Can you work these out from the model? Positions are in its coordinate system, mm. Coordinates: 2 decimals unless noted, no trailing zeros. Write each loop counter-clockwise with the first axis right and the second up, starting at its lowest first coordinate (ties: lowest second). Pieces come first, ordered by that corner, then holes. Notation, with made-up numbers: (-24.75, 36.25) -> (-17.75, 36.25) arc R28 ccw to (-17.75, 70.25) -> close; hole circle Ø2 at (32, 41). An arc over 180 degrees is marked (long way). Use one line per item in the form item = value.
```python
from build123d import *


with BuildPart() as part:
    # Sketch1 → Revolve1 (revolve)
    with BuildSketch(Plane(origin=(0, 0, 0), x_dir=(0, 0, -1), z_dir=(1, 0, 0)), mode=Mode.PRIVATE) as revolve1_sk:
        with BuildLine():
            Line((0.8, 49), (1.5, 49))
            Line((1.5, 49), (1.5, 46.5))
            Line((1.5, 46.5), (1.25, 46.5))
            Line((1.25, 46.5), (0, 46))
            Line((0, 46), (-1.25, 46.5))
            Line((-1.25, 46.5), (-1.5, 46.5))
            Line((-1.5, 46.5), (-1.5, 49))
            Line((-1.5, 49), (-0.8, 49))
            ThreePointArc((-0.8, 49), (0, 48.833030278), (0.8, 49))
        make_face()
    revolve(revolve1_sk.sketch.rotate(Axis((0, 0, 0), (0, 0, -1)), 90), axis=Axis((0, 0, 0), (0, 0, -1)))


solid = part.part
```
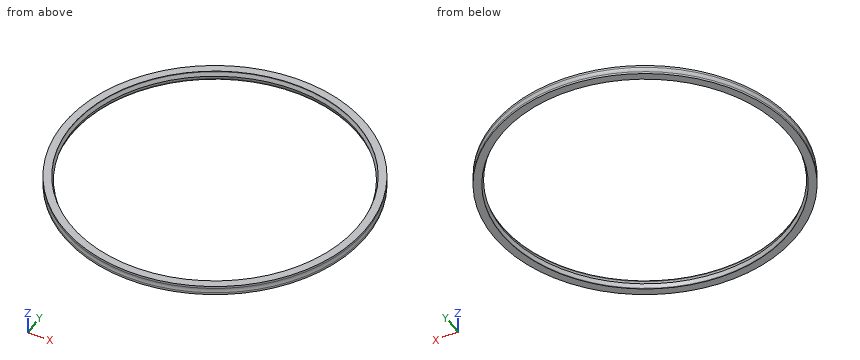
Q1. If I drill on line 1 (Y direction, x = 0, z = -1.25); line 2 (X direction, y = 9.5, z = 1.3); line 3 (Y direction, x = 15, z = -1.3), over which ranges is the centre line in solid material (lowest first)? Write a range as from..to.
Return value:
line_1 = -49..-46.5, 46.5..49
line_2 = -48.07..-45.52, 45.52..48.07
line_3 = -46.65..-44.01, 44.01..46.65
Q2. Will these pins go through, and if not, where does the flat tip stop? pin 1 (1 mm diameter, centred on y = 21.5, z = -1, fed in from +X); pin 2 (12 mm diameter, centred on x = 32, y = 28, fed in from +Z).
Return value:
pin_1 = 44.27
pin_2 = 1.5
Q3. Suppose I cut it at A-A (y = 0). Write out the boundary of the cut face in (x, z), then the cut area to 3 significant figures.
Return value:
outline = (-49, -1.5) -> (-46.5, -1.5) -> (-46.5, -1.25) -> (-46, 0) -> (-46.5, 1.25) -> (-46.5, 1.5) -> (-49, 1.5) -> (-49, 0.8) arc R2 cw to (-49, -0.8) -> close; (46, 0) -> (46.5, -1.25) -> (46.5, -1.5) -> (49, -1.5) -> (49, -0.8) arc R2 cw to (49, 0.8) -> (49, 1.5) -> (46.5, 1.5) -> (46.5, 1.25) -> close
area = 15.9 mm2
